The listing builds one solid part. Answer for the finished solid, in the listing's coordinates (mm). A direction names the side the tool comes from. Coordinates: 2 decimals unless noted, no trailing zeros. Order: outer loops, then holes, each group sorted by start corner. A loop starts at its lowest first (then second) coordinate and runs counter-clockwise, first axis right, second up. Notation, with made-up numbers: (-14, 27) -> (28, 27) arc R27 cw to (28, 66) -> close; hole circle Ø7 at (52.5, 89). An arc over 180 degrees is marked (long way). Return JSON: item names as keys, results as strings.
from build123d import *

# Parameters (mm, degrees)
F0_W          = 31.4
F0_H          = 31.4
F0_W_2        = 25.8
F0_H_2        = 25.8
F1_DEPTH      = 50.8
F1_DEPTH_BACK = 50.8
F2_W          = 28
F2_H          = 28
F3_DEPTH      = 3
F3_DEPTH_BACK = 3
F4_SIZE       = 12
F5_SIZE       = 2
F6_SIZE       = 2.6


with BuildPart() as f1:
    # F0 (on Top) → F1 (new body, two sides)
    with BuildSketch(Plane.XY) as f1_sk:
        Rectangle(F0_W, F0_H)
        Rectangle(F0_W_2, F0_H_2, mode=Mode.SUBTRACT)
    extrude(amount=F1_DEPTH)
    extrude(f1_sk.sketch, amount=-F1_DEPTH_BACK)

    # F2 (on Top) → F3 (join, two sides)
    with BuildSketch(Plane.XY) as f3_sk:
        Rectangle(F2_W, F2_H)
    extrude(amount=F3_DEPTH)
    extrude(f3_sk.sketch, amount=-F3_DEPTH_BACK)

    # F4
    f4_edges = [f1.edges().sort_by_distance(p)[0] for p in [
        (0, 12.9, 3),
        (12.9, 0, 3),
        (0, -12.9, 3),
        (-12.9, 0, 3),
    ]]
    chamfer(f4_edges, length=F4_SIZE)

    # F5
    f5_edges = [f1.edges().sort_by_distance(p)[0] for p in [
        (15.7, -15.7, 0),
        (-15.7, -15.7, 0),
        (15.7, 15.7, 0),
        (-15.7, 15.7, 0),
    ]]
    chamfer(f5_edges, length=F5_SIZE)

    # F6 (call 1 of 4: OpenCascade refuses the feature's edges together)
    f6_edges = [f1.edges().sort_by_distance(p)[0] for p in [
        (15.7, 0, -50.8),
    ]]
    chamfer(f6_edges, length=F6_SIZE)

    # F6#2 (call 2 of 4)
    f6_2_edges = [f1.edges().sort_by_distance(p)[0] for p in [
        (0, -15.7, -50.8),
    ]]
    chamfer(f6_2_edges, length=F6_SIZE)

    # F6#3 (call 3 of 4)
    f6_3_edges = [f1.edges().sort_by_distance(p)[0] for p in [
        (-15.7, 0, -50.8),
    ]]
    chamfer(f6_3_edges, length=F6_SIZE)

    # F6#4 (call 4 of 4)
    f6_4_edges = [f1.edges().sort_by_distance(p)[0] for p in [
        (0, 15.7, -50.8),
    ]]
    chamfer(f6_4_edges, length=F6_SIZE)


solid = f1.part
1. Consider line 1 (Y direction, x = 0, z = -6); line 2 (Z direction, x = -4.5, y = 7). Determine where each line is inside the solid, lowest interval first. Write a range as from..to.
Answer block:
{"line 1": "y = -15.7..-12.9, 12.9..15.7", "line 2": "z = -3..9.1"}
2. The part is cut by section A-A on z = 5. Give the vertices of the cut face in (x, y), and give its area (3 significant figures).
Answer block:
{"outline": "(-15.7, -13.7) -> (-13.7, -15.7) -> (13.7, -15.7) -> (15.7, -13.7) -> (15.7, 13.7) -> (13.7, 15.7) -> (-13.7, 15.7) -> (-15.7, 13.7) -> close; hole (-2.9, -2.9) -> (2.9, -2.9) -> (2.9, 2.9) -> (-2.9, 2.9) -> close", "area": "944 mm2"}
3. The part is cut by section D-D on z = -12.5. Give the vertices of the cut face in (x, y).
Answer block:
{"outline": "(-15.7, -13.7) -> (-13.7, -15.7) -> (13.7, -15.7) -> (15.7, -13.7) -> (15.7, 13.7) -> (13.7, 15.7) -> (-13.7, 15.7) -> (-15.7, 13.7) -> close; hole (-12.9, -12.9) -> (12.9, -12.9) -> (12.9, 12.9) -> (-12.9, 12.9) -> close"}
4. The part is cut by section B-B on x = 8. Give the vertices of the cut face in (y, z).
Answer block:
{"outline": "(-15.7, -48.2) -> (-13.1, -50.8) -> (-12.9, -50.8) -> (-12.9, -3) -> (12.9, -3) -> (12.9, -50.8) -> (13.1, -50.8) -> (15.7, -48.2) -> (15.7, 50.8) -> (12.9, 50.8) -> (12.9, 15) -> (8, 10.1) -> (-8, 10.1) -> (-12.9, 15) -> (-12.9, 50.8) -> (-15.7, 50.8) -> close"}
5. The part is cut by section C-C on y = 2.5. Give the vertices of the cut face in (x, z).
Answer block:
{"outline": "(-15.7, -48.2) -> (-13.1, -50.8) -> (-12.9, -50.8) -> (-12.9, -3) -> (12.9, -3) -> (12.9, -50.8) -> (13.1, -50.8) -> (15.7, -48.2) -> (15.7, 50.8) -> (12.9, 50.8) -> (12.9, 15) -> (2.5, 4.6) -> (-2.5, 4.6) -> (-12.9, 15) -> (-12.9, 50.8) -> (-15.7, 50.8) -> close"}
6. Determine the mould class of faces 1 (the face through (0, 12.9, -27)), 2 (the face through (-14.4, -0.2, -49.5)), 3 (the face through (0, 15.7, 2)) for opening direction Y: pulls with the +Y half, pulls with the -Y half, needs draft (parallel to the pull), parting line crosses it, or undercut.
Answer block:
{"face 1": "undercut", "face 2": "needs draft", "face 3": "pulls with the +Y half"}
7. Each of these flat-tipped pins is pushed along its axis until it touches: pin 1 Ø0.5 at (x, y) = (0.5, -0.5) entering from +Z; pin 2 Ø1 at (x, y) = (-10.5, -6) entering from +Z. Where does it stop, or does it pass through?
Answer block:
{"pin 1": "stops at z = 3", "pin 2": "stops at z = 13.1"}
8. For faces 4 (the face through (12.9, 0, 33)), 5 (the face through (-15.7, 0, 2)), 6 (the face through (0, -12.9, -27)), determine the directions among +Z, -Z, +X, -X, +Y, -Y from which every point of the face is accessible in a straight line to the end or side of a thin tool.
Answer block:
{"face 4": "+Z", "face 5": "+Z, -Z, -X, +Y, -Y", "face 6": "-Z"}
